The listing builds one solid part. Answer for the finished solid, in the listing's coordinates (mm). Face numbers are marked on the shaded views. A direction names the side the tool comes from. Coordinates: 2 decimals unless noted, no trailing zeros. Write each loop counter-clockwise with the first axis right and the second up, starting at its lowest first coordinate (ties: lowest second). Pieces come first, ordered by that corner, then holes. Notation, with made-up numbers: M 85.25,28.25 L 130.25,28.25 A24 ccw 130.25,66.25 Z; hole C 39.5,61.25 d7. An arc over 180 degrees is marked long. Write item = value, one per line. Start each with the question number.
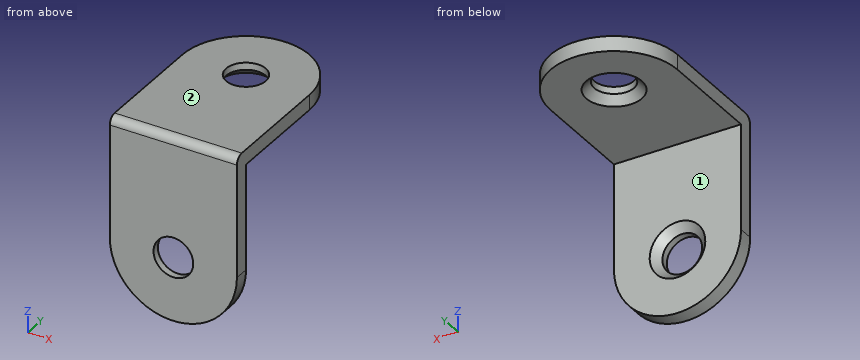
```python
from build123d import *

# Parameters (mm, degrees)
SKETCH_1_R      = 2.5
EXTRUDE_1_DEPTH = 1.9
SKETCH_3_R      = 2.5
EXTRUDE_2_DEPTH = 1.9
FILLET_1_R      = 1
CHAMFER_1_SIZE  = 1


with BuildPart() as part:
    # 草图1 → 凸台-拉伸1 (new body)
    with BuildSketch(Plane.XY):
        with BuildLine():
            Line((0, 15.076269086), (0, 0))
            Line((0, 0), (16, 0))
            Line((16, 0), (16, 15.076269086))
            ThreePointArc((16, 15.076269086), (8, 23.076269086), (0, 15.076269086))
        make_face()
        with Locations(Location((8, 15.076269086, 0), (0, 0, 180))):
            Circle(SKETCH_1_R, mode=Mode.SUBTRACT)
    extrude(amount=EXTRUDE_1_DEPTH)

    # 草图3 → 凸台-拉伸2 (add)
    with BuildSketch(Plane(origin=(0, 0, 0), x_dir=(1, 0, 0), z_dir=(0, 1, 0))):
        with BuildLine():
            Line((0, -1.9), (16, -1.9))
            Line((16, -1.9), (16, 13.272714332))
            ThreePointArc((16, 13.272714332), (8, 21.272714332), (0, 13.272714332))
            Line((0, 13.272714332), (0, -1.9))
        make_face()
        with Locations(Location((8, 13.272714332, 0), (0, 0, 90))):
            Circle(SKETCH_3_R, mode=Mode.SUBTRACT)
    extrude(amount=EXTRUDE_2_DEPTH)

    # 圆角1
    fillet_1_edges = [part.edges().sort_by_distance(p)[0] for p in [
        (8, 0, 1.9),
    ]]
    fillet(fillet_1_edges, radius=FILLET_1_R)

    # 倒角1
    chamfer_1_edges = [part.edges().sort_by_distance(p)[0] for p in [
        (8, 1.9, -10.772714332),
        (10.5, 15.076269086, 0),
    ]]
    chamfer(chamfer_1_edges, length=CHAMFER_1_SIZE)


solid = part.part
```
1. The part is cut by section B-B, the plane x = 2.75. Write down the section's boundary in (y, z).
2. Straight lines are drawn through the part: L1, parallel to Y at x = 13.25, z = -11.75; L2, parallel to Z at x = 8, y = 0.25. For each, find the intervals that lie inside material, in ascending order. Write a range as [from, to].
3. The part is cut by section A-A, the plane x = 8. Write down the section's boundary in (y, z).
4. The part is cut by section C-C, the plane z = -9.25. Write down the section's boundary in (x, y), and give its area (3 significant figures).
5. Each of these flat-tipped pins is pushed along its axis until it touches: pin 1 (5 mm diameter, centred on x = 10.5, z = -13.5, fed in from +Y); pin 2 (6 mm diameter, centred on x = 8, y = 15.08, fed in from -Z); pin 3 (2 mm diameter, centred on y = 3.5, z = -4, fed in from -X); pin 4 (8 mm diameter, centred on x = 9, y = 10, fed in from -Z). Where does it stop, or does it pass through?
6. For the marked faces 1 and 2, determine the directions among +Z, -Z, +X, -X, +Y, -Y from which every point of the face is accessible in a straight line to the end or side of a thin tool.
Solution:
q1.outline = M 0,-19.31 L 1.9,-19.31 L 1.9,0 L 21.11,0 L 21.11,1.9 L 1,1.9 A1 ccw 0,0.9 Z
q2.L1 = [0, 1.9]
q2.L2 = [-21.27, -15.77], [-10.77, 1.56]
q3.outline = M 0,-21.27 L 1.9,-21.27 L 1.9,-16.77 L 0.9,-15.77 L 0,-15.77 Z; M 0,-10.77 L 0.9,-10.77 L 1.9,-9.77 L 1.9,0 L 11.58,0 L 12.58,1 L 12.58,1.9 L 1,1.9 A1 ccw 0,0.9 Z; M 17.58,1 L 18.58,0 L 23.08,0 L 23.08,1.9 L 17.58,1.9 Z
q4.outline = M 0,0 L 16,0 L 16,1.9 L 0,1.9 Z
q4.area = 30.4 mm^2
q5.pin_1 = 1.9
q5.pin_2 = 0.5
q5.pin_3 = through
q5.pin_4 = 0
q6.face_1 = -Z, +X, -X, +Y
q6.face_2 = +Z, +X, -X, +Y, -Y
